Check sheet for the drawn part. Datum: minimum x, y, z corner. Units: mm. A direction names the side the tool comes from. Round coordinates to 2 decimals unless told otherwise and drop trailing zeros. Order: outer loops, then holes, each group sorted by start corner. A loop starts at its lowest first (then second) coordinate and runs counter-clockwise, first axis right, second up.
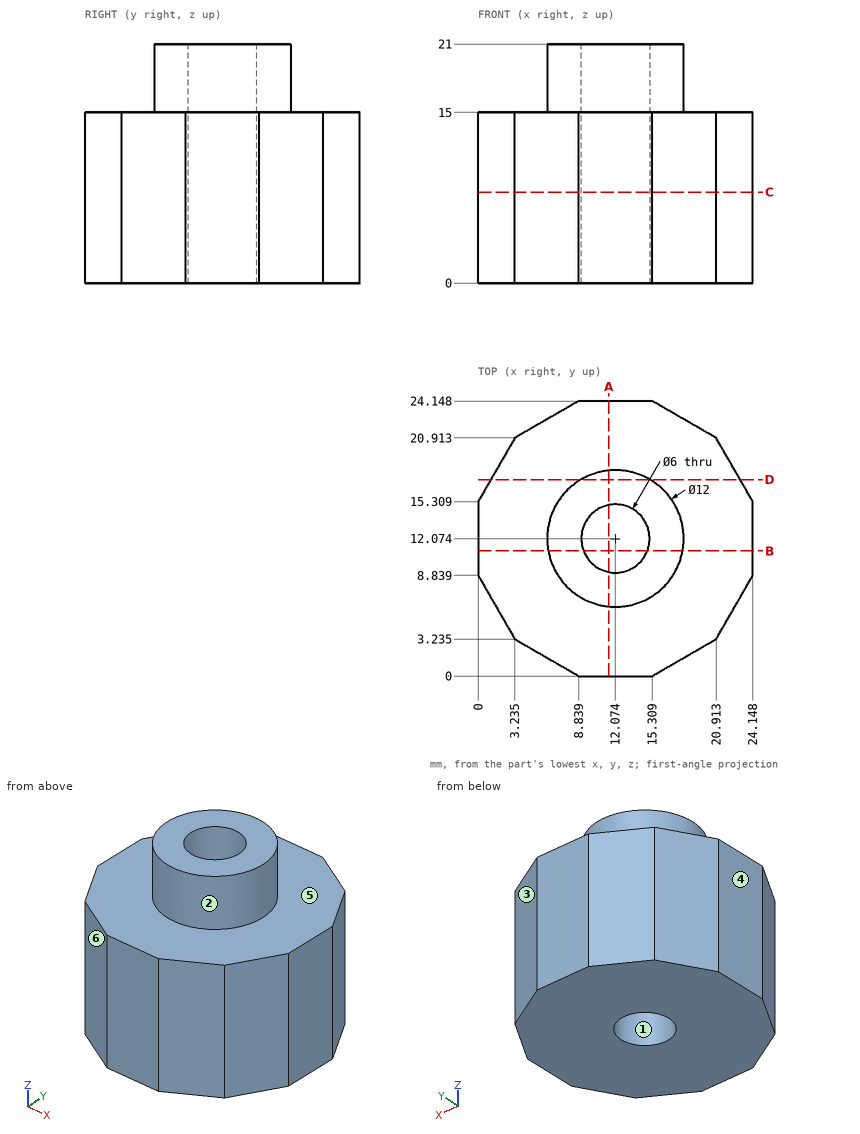
1) Sectioned sample at B-B on y = 11. Record the cut outline in (x, z) (1 decimal).
2) Gauge pin test, flat ends, axial feed: pin 1 (1 mm diameter, centred on y = 20.5, z = 5, fed in from +X); pin 2 (8 mm diameter, centred on x = 21.5, z = 5.5, fed in from +Y); pin 3 (2 mm diameter, centred on y = 21.5, z = 4, fed in from -X). Record the tip position at first contact, or that the pin passes through.
3) Sectioned sample at A-A on x = 11.5. Record the cut outline in (y, z), and give its area (3 significant figures).
4) Sectioned sample at C-C on z = 8. Record the cut outline in (x, y) (1 decimal).
5) Set-up check for the marked faces 5 and 6: record each of +Z, -Z, +X, -X, +Y, -Y from which the full face is reachable in a straight line by a thin tool's end or side.
6) Draft check along X on the marked faces 1, 2, 3 and 4. Enter one of: pulls with the +X half, pulls with the -X half, needs draft (parallel to the pull), parting line crosses it, or undercut.
7) Sectioned sample at D-D on y = 17.25. Record the cut outline in (x, z), and give its area (3 significant figures).
8) Scan lines: line 1 (X direction, y = 12.25, z = 8.25); line 2 (Z direction, x = 9.25, y = 5.5); line 3 (Y direction, x = 12, z = 7) (1 decimal). Record each from-to range of solid material in increasing order.
Values found:
1. outline: (0, 0) - (9.3, 0) - (9.3, 21) - (6.2, 21) - (6.2, 15) - (0, 15) - close; (14.9, 0) - (24.1, 0) - (24.1, 15) - (18, 15) - (18, 21) - (14.9, 21) - close
2. pin 1: stops at x = 21.44
2. pin 2: stops at y = 22.88
2. pin 3: stops at x = 3
3. outline: (0, 0) - (9.13, 0) - (9.13, 21) - (6.1, 21) - (6.1, 15) - (0, 15) - close; (15.02, 0) - (24.15, 0) - (24.15, 15) - (18.05, 15) - (18.05, 21) - (15.02, 21) - close
3. area: 310 mm2
4. outline: (0, 8.8) - (3.2, 3.2) - (8.8, 0) - (15.3, 0) - (20.9, 3.2) - (24.1, 8.8) - (24.1, 15.3) - (20.9, 20.9) - (15.3, 24.1) - (8.8, 24.1) - (3.2, 20.9) - (0, 15.3) - close; hole circle Ø6 at (12.1, 12.1)
5. face 5: +Z
5. face 6: +Z, -Z, -X, -Y
6. face 1: undercut
6. face 2: parting line crosses it
6. face 3: pulls with the +X half
6. face 4: pulls with the -X half
7. outline: (1.12, 0) - (23.03, 0) - (23.03, 15) - (15.11, 15) - (15.11, 21) - (9.04, 21) - (9.04, 15) - (1.12, 15) - close
7. area: 365 mm2
8. line 1: x = 0 to 9.08, 15.07 to 24.15
8. line 2: z = 0 to 15
8. line 3: y = 0 to 9.1, 15.1 to 24.1
